Design review of the part built by this model. Coordinates are the model's own, in mm. A direction names the side the tool comes from. Give positions to 0.01 mm unless a question says otherwise; leave off trailing zeros. Loops run counter-clockwise (first coordinate to the right, second up) from the corner with the lowest first, then second, coordinate; pieces in that order, holes last. Notation, with made-up numbers: (1.25, 6.5) - (26.25, 6.5) arc R17 cw to (26.25, 15.5) - close; hole circle Ø1 at (13.25, 64.5). An arc over 180 degrees is marked (long way). Write each question's results on one line, items separated by ' | '.
from build123d import *

# Parameters (mm, degrees)
BOSS_EXTRUDE1_DEPTH             = 4
SKETCH3_W                       = 7.1
SKETCH3_H                       = 8
BOSS_EXTRUDE3_DEPTH             = 3
SKETCH4_R                       = 2.05
CUT_EXTRUDE1_DEPTH              = 7
MIRROR2_COPY_1_SKETCH_W         = 7.1
MIRROR2_COPY_1_SKETCH_H         = 8
MIRROR2_COPY_1_DEPTH            = 3
MIRROR2_COPY_2_SKETCH_R         = 2.05
MIRROR2_COPY_2_DEPTH            = 7
SKETCH5_W                       = 60
SKETCH5_H                       = 9
CUT_EXTRUDE2_DEPTH              = 76.4917214
FILLET1_R                       = 2
SKETCH7_W                       = 111.8
SKETCH7_H                       = 1
CUT_EXTRUDE3_DEPTH              = 76.4917214
SKETCH8_W                       = 126
SKETCH8_H                       = 2
BOSS_EXTRUDE4_DEPTH             = 38
SKETCH9_W                       = 12
SKETCH9_H                       = 18
CUT_EXTRUDE4_DEPTH              = 10
SKETCH10_W                      = 7.1
SKETCH10_H                      = 4
BOSS_EXTRUDE5_DEPTH             = 3
SKETCH12_W                      = 1.5
SKETCH12_H                      = 4
BOSS_EXTRUDE6_DEPTH             = 2
SKETCH13_W                      = 40
SKETCH13_H                      = 2
BOSS_EXTRUDE7_DEPTH             = 38
SKETCH14_W                      = 1.5
SKETCH14_H                      = 4
BOSS_EXTRUDE8_DEPTH             = 1
BOSS_EXTRUDE9_REACH             = 85.744
BOSS_EXTRUDE9_DIRECTION_2_REACH = 85.744
SKETCH16_W                      = 20
SKETCH16_H                      = 14
SKETCH16_W_2                    = 14.5
SKETCH16_H_2                    = 9
BOSS_EXTRUDE10_DEPTH            = 4
SKETCH17_W                      = 12
SKETCH17_H                      = 18
CUT_EXTRUDE5_DEPTH              = 84.743656476
SKETCH18_W                      = 6
SKETCH18_H                      = 6
CUT_EXTRUDE6_DEPTH              = 86.632937588
SKETCH22_R                      = 1.25
CUT_EXTRUDE7_DEPTH              = 4
SKETCH25_W                      = 6
SKETCH25_H                      = 38
CUT_EXTRUDE11_DEPTH             = 10
SKETCH26_W                      = 5.701552738
SKETCH26_H                      = 30.562488548
SKETCH26_W_2                    = 6.53419365
SKETCH26_H_2                    = 28.524331859
CUT_EXTRUDE12_DEPTH             = 85.498520697
CUT_EXTRUDE12_DEPTH_BACK        = 85.498520697
SKETCH27_R                      = 1.25
CUT_EXTRUDE13_DEPTH             = 86.632937588
SKETCH28_W                      = 99.8
SKETCH28_H                      = 0.6
SKETCH28_W_2                    = 87.8
CUT_EXTRUDE14_DEPTH             = 86.632937588


with BuildPart() as part:
    # Sketch1 → Boss-Extrude1 (new body)
    with BuildSketch(Plane(origin=(0, 0, 0), x_dir=(1, 0, 0), z_dir=(0, 1, 0))):
        Polygon((-63, -34), (-55.9, -34), (-55.9, -41), (55.9, -41), (55.9, -34), (63, -34), (63, 34), (55.9, 34), (55.9, 41), (-55.9, 41), (-55.9, 34), (-63, 34), align=None)
    extrude(amount=BOSS_EXTRUDE1_DEPTH)

    # Sketch3 → Boss-Extrude3 (add)
    with BuildSketch(Plane.XZ):
        with Locations((-59.45, -30)):
            Rectangle(SKETCH3_W, SKETCH3_H)
    boss_extrude3 = extrude(amount=BOSS_EXTRUDE3_DEPTH)

    # Sketch4 → Cut-Extrude1 (cut)
    with BuildSketch(Plane(origin=(0, 0, -34), x_dir=(-1, 0, 0), z_dir=(0, 0, -1))):
        with Locations((59.45, 0.5)):
            Circle(SKETCH4_R)
    cut_extrude1 = extrude(amount=-CUT_EXTRUDE1_DEPTH, mode=Mode.SUBTRACT)

    # Mirror1: Boss-Extrude3, Cut-Extrude1 across plane
    add(boss_extrude3.mirror(Plane(origin=(0, 0, 0), x_dir=(0, 0, 1), z_dir=(1, 0, 0))))
    add(cut_extrude1.mirror(Plane(origin=(0, 0, 0), x_dir=(0, 0, 1), z_dir=(1, 0, 0))), mode=Mode.SUBTRACT)

    # Mirror2: Boss-Extrude3, Cut-Extrude1 across plane
    add(boss_extrude3.mirror(Plane.XY))
    add(cut_extrude1.mirror(Plane.XY), mode=Mode.SUBTRACT)

    # Mirror2 copy 1 sketch → Mirror2 copy 1 (add)
    with BuildSketch(Plane(origin=(0, 0, 0), x_dir=(-1, 0, 0), z_dir=(0, -1, 0))):
        with Locations((-59.45, -30)):
            Rectangle(MIRROR2_COPY_1_SKETCH_W, MIRROR2_COPY_1_SKETCH_H)
    extrude(amount=MIRROR2_COPY_1_DEPTH)

    # Mirror2 copy 2 sketch → Mirror2 copy 2 (cut)
    with BuildSketch(Plane.XY.offset(34)):
        with Locations((59.45, 0.5)):
            Circle(MIRROR2_COPY_2_SKETCH_R)
    extrude(amount=-MIRROR2_COPY_2_DEPTH, mode=Mode.SUBTRACT)

    # Sketch5 → Cut-Extrude2 (cut, through all)
    with BuildSketch(Plane(origin=(0, 4, 0), x_dir=(1, 0, 0), z_dir=(0, 1, 0))):
        with Locations((0, 33.5)):
            Rectangle(SKETCH5_W, SKETCH5_H)
    extrude(amount=-CUT_EXTRUDE2_DEPTH, mode=Mode.SUBTRACT)

    # Fillet1
    fillet1_edges = [part.edges().sort_by_distance(p)[0] for p in [
        (-30, 2, -29),
        (-30, 2, -38),
        (30, 2, -38),
        (30, 2, -29),
    ]]
    fillet(fillet1_edges, radius=FILLET1_R)

    # Sketch7 → Cut-Extrude3 (cut, through all)
    with BuildSketch(Plane(origin=(0, 4, 0), x_dir=(1, 0, 0), z_dir=(0, 1, 0))):
        with Locations((0, 40.5)):
            Rectangle(SKETCH7_W, SKETCH7_H)
        with Locations((0, -40.5)):
            Rectangle(SKETCH7_W, SKETCH7_H)
    extrude(amount=-CUT_EXTRUDE3_DEPTH, mode=Mode.SUBTRACT)

    # Sketch8 → Boss-Extrude4 (add)
    with BuildSketch(Plane.XZ):
        with Locations((0, 21)):
            Rectangle(SKETCH8_W, SKETCH8_H)
    extrude(amount=BOSS_EXTRUDE4_DEPTH)

    # Sketch9 → Cut-Extrude4 (cut)
    with BuildSketch(Plane(origin=(0, 4, 0), x_dir=(1, 0, 0), z_dir=(0, 1, 0))):
        with Locations((-49.9, -31)):
            Rectangle(SKETCH9_W, SKETCH9_H)
    extrude(amount=-CUT_EXTRUDE4_DEPTH, mode=Mode.SUBTRACT)

    # Sketch10 → Boss-Extrude5 (add)
    with BuildSketch(Plane.XZ.offset(3)):
        with Locations((-59.45, 24)):
            Rectangle(SKETCH10_W, SKETCH10_H)
        with Locations((59.45, 24)):
            Rectangle(SKETCH10_W, SKETCH10_H)
    extrude(amount=-BOSS_EXTRUDE5_DEPTH)

    # Sketch12 → Boss-Extrude6 (add)
    with BuildSketch(Plane.ZY.offset(56)):
        Polygon((22, -5.8), (22, -16.2), (24.7, -13.5), (24.7, -8.5), align=None)
        with Locations((23.35, -11)):
            Rectangle(SKETCH12_W, SKETCH12_H, mode=Mode.SUBTRACT)
        Polygon((22, -20.8), (22, -31.2), (24.7, -28.5), (24.7, -23.5), align=None)
        with Locations((23.35, -26)):
            Rectangle(SKETCH12_W, SKETCH12_H, mode=Mode.SUBTRACT)
    boss_extrude6 = extrude(amount=-BOSS_EXTRUDE6_DEPTH)

    # Mirror3: Boss-Extrude6 across plane
    add(boss_extrude6.mirror(Plane(origin=(-49.9, 0, 0), x_dir=(0, 0, 1), z_dir=(1, 0, 0))))

    # Sketch13 → Boss-Extrude7 (add)
    with BuildSketch(Plane.XZ):
        with Locations((0, -20.5)):
            Rectangle(SKETCH13_W, SKETCH13_H)
    extrude(amount=BOSS_EXTRUDE7_DEPTH)

    # Sketch14 → Boss-Extrude8 (add, symmetric)
    with BuildSketch(Plane(origin=(0, 0, 0), x_dir=(0, 0, -1), z_dir=(1, 0, 0))):
        Polygon((24.2, -8.5), (21.5, -5.8), (21.5, -16.2), (24.2, -13.5), align=None)
        with Locations((22.85, -11)):
            Rectangle(SKETCH14_W, SKETCH14_H, mode=Mode.SUBTRACT)
        Polygon((24.2, -28.5), (24.2, -23.5), (21.5, -20.8), (21.5, -31.2), align=None)
        with Locations((22.85, -26)):
            Rectangle(SKETCH14_W, SKETCH14_H, mode=Mode.SUBTRACT)
    extrude(amount=BOSS_EXTRUDE8_DEPTH, both=True)

    # Boss-Extrude9: up to this face of the body (flat: up to its plane)
    boss_extrude9_end = Plane(part.part.faces().sort_by_distance((-20, -19, -20.5))[0])
    # Sketch15 → Boss-Extrude9 (add, up to the picked face)
    with BuildSketch(Plane(origin=(0, 0, 0), x_dir=(0, 0, -1), z_dir=(1, 0, 0)), mode=Mode.PRIVATE) as boss_extrude9_sk1:
        Polygon((19.5, 0), (19.5, -5), (16.613248654, 0), align=None)
    boss_extrude9_tool1 = split(extrude(boss_extrude9_sk1.sketch, amount=-BOSS_EXTRUDE9_REACH, mode=Mode.PRIVATE), bisect_by=boss_extrude9_end, keep=Keep.BOTH, mode=Mode.PRIVATE)
    add(boss_extrude9_tool1.solids().sort_by(Axis((0, -1.666667, -18.53775), (-1, 0, 0)))[0])

    # Boss-Extrude9 direction 2: up to this face of the body (flat: up to its plane)
    boss_extrude9_direction_2_end = Plane(part.part.faces().sort_by_distance((20, -19, -20.5))[0])
    # Sketch15 → Boss-Extrude9 direction 2 (add, up to the picked face)
    with BuildSketch(Plane(origin=(0, 0, 0), x_dir=(0, 0, -1), z_dir=(1, 0, 0)), mode=Mode.PRIVATE) as boss_extrude9_direction_2_sk1:
        Polygon((19.5, 0), (19.5, -5), (16.613248654, 0), align=None)
    boss_extrude9_direction_2_tool1 = split(extrude(boss_extrude9_direction_2_sk1.sketch, amount=BOSS_EXTRUDE9_DIRECTION_2_REACH, mode=Mode.PRIVATE), bisect_by=boss_extrude9_direction_2_end, keep=Keep.BOTH, mode=Mode.PRIVATE)
    add(boss_extrude9_direction_2_tool1.solids().sort_by(Axis((0, -1.666667, -18.53775), (1, 0, 0)))[0])

    # Sketch16 → Boss-Extrude10 (add)
    with BuildSketch(Plane.XY.offset(40)):
        with Locations((30, -7)):
            Rectangle(SKETCH16_W, SKETCH16_H)
        with Locations((30, -7)):
            Rectangle(SKETCH16_W_2, SKETCH16_H_2, mode=Mode.SUBTRACT)
    extrude(amount=-BOSS_EXTRUDE10_DEPTH)

    # Sketch17 → Cut-Extrude5 (cut, through all)
    with BuildSketch(Plane.XZ):
        with Locations((49.9, 31)):
            Rectangle(SKETCH17_W, SKETCH17_H)
    extrude(amount=-CUT_EXTRUDE5_DEPTH, mode=Mode.SUBTRACT)

    # Sketch18 → Cut-Extrude6 (cut, through all)
    with BuildSketch(Plane(origin=(0, 4, 0), x_dir=(1, 0, 0), z_dir=(0, 1, 0))):
        with Locations((52.9, 37)):
            Rectangle(SKETCH18_W, SKETCH18_H)
        with Locations((-52.9, 37)):
            Rectangle(SKETCH18_W, SKETCH18_H)
    extrude(amount=-CUT_EXTRUDE6_DEPTH, mode=Mode.SUBTRACT)

    # Sketch22 → Cut-Extrude7 (cut)
    with BuildSketch(Plane(origin=(0, 4, 0), x_dir=(1, 0, 0), z_dir=(0, 1, 0))):
        with Locations(Location((31, 25, 0), (0, 0, 270))):
            Circle(SKETCH22_R)
        with Locations(Location((-31, -17, 0), (0, 0, 270))):
            Circle(SKETCH22_R)
    extrude(amount=-CUT_EXTRUDE7_DEPTH, mode=Mode.SUBTRACT)

    # Sketch25 → Cut-Extrude11 (cut)
    with BuildSketch(Plane(origin=(0, 0, -21.5), x_dir=(-1, 0, 0), z_dir=(0, 0, -1))):
        with Locations((-17, -19)):
            Rectangle(SKETCH25_W, SKETCH25_H)
        with Locations((17, -19)):
            Rectangle(SKETCH25_W, SKETCH25_H)
    extrude(amount=-CUT_EXTRUDE11_DEPTH, mode=Mode.SUBTRACT)

    # Sketch26 → Cut-Extrude12 (cut, two sides)
    with BuildSketch(Plane.ZY.offset(1)) as cut_extrude12_sk:
        with Locations((-24.350776369, -21.081244274)):
            Rectangle(SKETCH26_W, SKETCH26_H)
        with Locations((25.267096825, -20.06216593)):
            Rectangle(SKETCH26_W_2, SKETCH26_H_2)
    extrude(amount=CUT_EXTRUDE12_DEPTH, mode=Mode.SUBTRACT)
    extrude(cut_extrude12_sk.sketch, amount=-CUT_EXTRUDE12_DEPTH_BACK, mode=Mode.SUBTRACT)

    # Sketch27 → Cut-Extrude13 (cut, through all)
    with BuildSketch(Plane(origin=(0, 4, 0), x_dir=(1, 0, 0), z_dir=(0, 1, 0))):
        with Locations(Location((-33.2, 26.5, 0), (0, 0, 270))):
            Circle(SKETCH27_R)
        with Locations(Location((-33.2, -30.5, 0), (0, 0, 270))):
            Circle(SKETCH27_R)
        with Locations(Location((38.8, -30.5, 0), (0, 0, 270))):
            Circle(SKETCH27_R)
        with Locations(Location((38.8, 26.5, 0), (0, 0, 270))):
            Circle(SKETCH27_R)
    extrude(amount=-CUT_EXTRUDE13_DEPTH, mode=Mode.SUBTRACT)

    # Sketch28 → Cut-Extrude14 (cut, through all)
    with BuildSketch(Plane(origin=(0, 4, 0), x_dir=(1, 0, 0), z_dir=(0, 1, 0))):
        with Locations((0, 39.7)):
            Rectangle(SKETCH28_W, SKETCH28_H)
        with Locations((0, -39.7)):
            Rectangle(SKETCH28_W_2, SKETCH28_H)
    extrude(amount=-CUT_EXTRUDE14_DEPTH, mode=Mode.SUBTRACT)


solid = part.part
(1) Take a section at D-D on y = -30. Give the boundary of the cut face in (x, z), plus the area to 3 significant figures.
Answers below:
outline: (-63, 20) - (63, 20) - (63, 22) - (-63, 22) - close; (-14, -21.5) - (14, -21.5) - (14, -19.5) - (-14, -19.5) - close | area: 308 mm2
(2) Tool access review of faces 1 (the cylindrical face through (-57.4, 0.59, -30.55)), 2 (the flat face through (59, -3, 28)), 3 (the flat face through (61.1, -1, 34)), 4 (the flat face through (-55.9, -1, -30)), 5 (the flat face through (-43.9, 2, 31)): name each direction out of +Z, -Z, +X, -X, +Y, -Y from which nothing blocks a thin tool from reaching the whole face with its end or side.
Answers below:
face 1: -Z | face 2: +Z, +X, -X, -Y | face 3: +Z, +X, +Y, -Y | face 4: -Z, -Y | face 5: +Z, +Y, -Y
(3) Take a section at C-C on y = -9. Give the boundary of the cut face in (x, z).
Answers below:
outline: (-63, 20) - (63, 20) - (63, 22) - (-63, 22) - close; (-14, -21.5) - (14, -21.5) - (14, -19.5) - (-14, -19.5) - close; (20, 36) - (22.75, 36) - (22.75, 39.4) - (20, 39.4) - close; (37.25, 36) - (40, 36) - (40, 39.4) - (37.25, 39.4) - close
(4) Wall thickness on line 1 along Z through (x, y) = (-17, 2); line 2 along X through (y, z) = (1, -26); line 3 along Z through (x, y) = (-3.5, -13.5): over which ranges is each line inside the solid? List them lowest first. Write a range as from..to.
Answers below:
line 1: -39.4..-38, -29..39.4 | line 2: -63..-34.35, -32.05..30.25, 31.75..37.65, 39.95..63 | line 3: -21.5..-19.5, 20..22
(5) Insertion check: P1, Ø2, axis at x = 14.5, y = -4, coming from the -Z side; P2, Ø12, axis at x = 31.5, z = 2, coming from the -Y side; P3, Ø1, axis at y = -8, z = 38, coming from the +X side. Each pin has a flat end and moves straight along its axis. Give the tip position at first contact, or say it passes through.
Answers below:
P1: z = -21.5 | P2: y = 0 | P3: x = 40
(6) Take a section at A-A on z = 30.5. Give the boundary of the cut face in (x, y).
Answers below:
outline: (-63, -3) - (-55.9, -3) - (-55.9, 4) - (-63, 4) - close; (-43.9, 0) - (-34.45, 0) - (-34.45, 4) - (-43.9, 4) - close; (-31.95, 0) - (37.55, 0) - (37.55, 4) - (-31.95, 4) - close; (40.05, 0) - (43.9, 0) - (43.9, 4) - (40.05, 4) - close; (55.9, -3) - (63, -3) - (63, 4) - (55.9, 4) - close; hole circle Ø4.1 at (-59.45, 0.5); hole circle Ø4.1 at (59.45, 0.5)
(7) Draft analysis for pull direction X (two halves, no side actions). For faces 6 (the flat face through (-49.9, 2, -37)), 7 (the flat face through (0, -19, -21.5)), 8 (the flat face through (14, -19, -20)), 9 (the flat face through (0, 2, -29)), state which applies: pulls with the +X half, pulls with the -X half, needs draft (parallel to the pull), parting line crosses it, or undercut.
Answers below:
face 6: pulls with the -X half | face 7: needs draft | face 8: pulls with the +X half | face 9: undercut
(8) Take a section at B-B on x = -20. Give the boundary of the cut face in (y, z).
Answers below:
outline: (-38, 20) - (0, 20) - (0, -29) - (4, -29) - (4, 39.4) - (0, 39.4) - (0, 22) - (-38, 22) - close; (0, -39.4) - (4, -39.4) - (4, -38) - (0, -38) - close
